from build123d import *

# Parameters (mm, degrees)
CHAMFER1_SIZE = 1


with BuildPart() as part:
    # Sketch1 → Revolve1 (revolve)
    with BuildSketch(Plane(origin=(0, 0, 0), x_dir=(0, 0, -1), z_dir=(1, 0, 0))):
        with BuildLine():
            ThreePointArc((22.775, 24), (12.275, 13.5), (22.775, 3))
            Line((22.775, 3), (22.775, 0))
            Line((22.775, 0), (7.775, 0))
            Line((7.775, 0), (7.775, 27))
            Line((7.775, 27), (22.775, 27))
            Line((22.775, 27), (22.775, 24))
        make_face()
    revolve(axis=Axis((0, 0, 0), (0, 1, 0)))

    # Chamfer1
    # the kernel refuses this chamfer: 1 mm, written as the material it takes off along each edge
    with BuildSketch(Plane(origin=(0, 3, 0), x_dir=(0, 0, -1), z_dir=(1, 0, 0))) as chamfer1_piece_1:
        with BuildLine():
            Line((21.722073557, 0.052926443), (22.775, -CHAMFER1_SIZE))
            Line((22.775, -CHAMFER1_SIZE), (22.775, 0))
            ThreePointArc((22.775, 0), (22.233019365, 0.013997092), (21.722073557, 0.052926443))
        make_face()
    revolve(axis=Axis((0, 3, 0), (0, 1, 0)), mode=Mode.SUBTRACT)
    with BuildSketch(Plane(origin=(0, 0, 0), x_dir=(0, 0, -1), z_dir=(1, 0, 0))) as chamfer1_piece_2:
        Polygon((22.775, CHAMFER1_SIZE), (22.775 - CHAMFER1_SIZE, 0), (22.775, 0), align=None)
    revolve(axis=Axis((0, 0, 0), (0, 1, 0)), mode=Mode.SUBTRACT)
    with BuildSketch(Plane(origin=(0, 0, 0), x_dir=(0, 0, -1), z_dir=(1, 0, 0))) as chamfer1_piece_3:
        Polygon((7.775 + CHAMFER1_SIZE, 0), (7.775, CHAMFER1_SIZE), (7.775, 0), align=None)
    revolve(axis=Axis((0, 0, 0), (0, 1, 0)), mode=Mode.SUBTRACT)
    with BuildSketch(Plane(origin=(0, 27, 0), x_dir=(0, 0, -1), z_dir=(1, 0, 0))) as chamfer1_piece_4:
        Polygon((7.775, -CHAMFER1_SIZE), (7.775 + CHAMFER1_SIZE, 0), (7.775, 0), align=None)
    revolve(axis=Axis((0, 27, 0), (0, 1, 0)), mode=Mode.SUBTRACT)
    with BuildSketch(Plane(origin=(0, 27, 0), x_dir=(0, 0, -1), z_dir=(1, 0, 0))) as chamfer1_piece_5:
        Polygon((22.775 - CHAMFER1_SIZE, 0), (22.775, -CHAMFER1_SIZE), (22.775, 0), align=None)
    revolve(axis=Axis((0, 27, 0), (0, 1, 0)), mode=Mode.SUBTRACT)
    with BuildSketch(Plane(origin=(0, 24, 0), x_dir=(0, 0, -1), z_dir=(1, 0, 0))) as chamfer1_piece_6:
        with BuildLine():
            Line((21.722073557, -0.052926443), (22.775, CHAMFER1_SIZE))
            Line((22.775, CHAMFER1_SIZE), (22.775, 0))
            ThreePointArc((22.775, 0), (22.233019365, -0.013997092), (21.722073557, -0.052926443))
        make_face()
    revolve(axis=Axis((0, 24, 0), (0, 1, 0)), mode=Mode.SUBTRACT)


solid = part.part
Can you work these out from the model? Positions are in its coordinate system, mm. Give positions to 0.01 mm unless a question says otherwise; leave off trailing zeros. Order: outer loops, then holes, each group sorted by start corner. A loop starts at its lowest first (then second) coordinate and runs counter-clockwise, first axis right, second up. Notation, with made-up numbers: M 30,21 L 65,21 A22 cw 65,45 Z; hole C 78.5,68 d4. An arc over 180 degrees is marked long. Use one line per item in the form item = value.
Item 1: Thinking about a two-plate mould opening in Z: for faces 1 (the cylindrical face through (13.86, 25.49, 18.07)), 2 (the cylindrical face through (7.59, 13.68, 1.69)), 3 (the flat face through (0, 27, 9)), which applies, pulls with the +Z half, pulls with the -Z half, needs draft (parallel to the pull), parting line crosses it, or undercut?
Values follow:
face_1 = parting line crosses it
face_2 = undercut
face_3 = needs draft
Item 2: If we section it at C-C, the plane y = 11: Write out the boundary of the cut face in (x, z) (3 decimals), and give its area (3 significant figures).
Values follow:
outline = C 0,0 d25.154; hole C 0,0 d15.55
area = 307 mm^2
Item 3: If we section it at A-A, the plane z = 0: Write out the boundary of the cut face in (x, y) (3 decimals).
Values follow:
outline = M -22.775,1 L -21.775,0 L -8.775,0 L -7.775,1 L -7.775,26 L -8.775,27 L -21.775,27 L -22.775,26 L -22.775,25 L -21.722,23.947 A10.5 cw -21.722,3.053 L -22.775,2 Z; M 7.775,1 L 8.775,0 L 21.775,0 L 22.775,1 L 22.775,2 L 21.722,3.053 A10.5 cw 21.722,23.947 L 22.775,25 L 22.775,26 L 21.775,27 L 8.775,27 L 7.775,26 Z
Item 4: Will these pins go through, and if not, where does the flat tip stop? pin 1 Ø1.5 at (x, y) = (9, 21) entering from -Z; pin 2 Ø8 at (x, z) = (4, 2.5) entering from -Y; pin 3 Ø1 at (x, y) = (-7, 14) entering from -Z.
Values follow:
pin_1 = -13.67
pin_2 = 0.06
pin_3 = -10.43
Item 5: If I drill on line 1 along Y through (x, z) = (15, 7); line 2 along Y through (x, z) = (19, 8); line 3 along X through (y, z) = (14.75, 4), over which ranges is the centre line in solid material (lowest first)? Write a range as [from, to].
Values follow:
line_1 = [0, 5.04], [21.96, 27]
line_2 = [0, 3.22], [23.78, 27]
line_3 = [-11.68, -6.67], [6.67, 11.68]
Item 6: If we section it at B-B, the plane x = 0: Write out the boundary of the cut face in (y, z) (3 decimals).
Values follow:
outline = M 0,-21.775 L 1,-22.775 L 2,-22.775 L 3.053,-21.722 A10.5 cw 23.947,-21.722 L 25,-22.775 L 26,-22.775 L 27,-21.775 L 27,-8.775 L 26,-7.775 L 1,-7.775 L 0,-8.775 Z; M 0,8.775 L 1,7.775 L 26,7.775 L 27,8.775 L 27,21.775 L 26,22.775 L 25,22.775 L 23.947,21.722 A10.5 cw 3.053,21.722 L 2,22.775 L 1,22.775 L 0,21.775 Z
